```python
from build123d import *

# Parameters (mm, degrees)
F1_DEPTH  = 500
F2_W      = 73.9309489727
F2_H      = 500
F2_H_2    = 305.1662445068
F2_H_3    = 304.9542307854
F3_DEPTH  = 25.4
F4_R      = 5.11898469
F5_DEPTH  = 50.8
F6_R      = 82.2041903744
F6_R_2    = 5.11898469
F7_DEPTH  = 25.4
F8_R      = 5.8344538593
F9_DEPTH  = 50.8
F10_R     = 76.2
F11_DEPTH = 25.4
F12_R     = 6.35
F13_DEPTH = 50.8
F14_R     = 304.8
F14_R_2   = 6.35
F15_DEPTH = 25.4
F16_R     = 6.35
F17_DEPTH = 50.8


with BuildPart() as f1:
    # F0 (on Front) → F1 (new body)
    with BuildSketch(Plane.XZ):
        Polygon((-775.8201853523, 304.8), (-775.8201853523, 0), (500, 0), (500, 500), (0, 500), align=None)
    extrude(amount=F1_DEPTH)

    # F2 (on face) → F3 (join)
    with BuildSketch(Plane(origin=(0, 0, 0), x_dir=(1, 0, 0), z_dir=(0, 0, -1))):
        with Locations((-436.6519004107, 250)):
            Rectangle(F2_W, F2_H)
        with Locations((-436.6519004107, 652.5831222534)):
            Rectangle(F2_W, F2_H_2)
        with Locations((-436.6519004107, -152.4771153927)):
            Rectangle(F2_W, F2_H_3)
    extrude(amount=F3_DEPTH)

    # F4 (on face) → F5 (join)
    with BuildSketch(Plane.XZ.offset(805.1662445068)):
        with Locations((-437.0749592781, -14.6776270121)):
            Circle(F4_R)
    extrude(amount=F5_DEPTH)

    # F6 (on face) → F7 (join)
    with BuildSketch(Plane.XZ.offset(855.9662445068)):
        with Locations((-437.0749592781, -14.6776270121)):
            Circle(F6_R)
        with Locations((-437.0749592781, -14.6776270121)):
            Circle(F6_R_2, mode=Mode.SUBTRACT)
    extrude(amount=-F7_DEPTH)

    # F8 (on face) → F9 (join)
    with BuildSketch(Plane(origin=(0, 304.9542307854, 0), x_dir=(-1, 0, 0), z_dir=(0, 1, 0))):
        with Locations((435.6042742729, -14.3710989505)):
            Circle(F8_R)
    extrude(amount=F9_DEPTH)

    # F10 (on face) → F11 (join)
    with BuildSketch(Plane(origin=(0, 355.7542307854, 0), x_dir=(-1, 0, 0), z_dir=(0, 1, 0))):
        with Locations((435.6042742729, -14.3710989505)):
            Circle(F10_R)
    extrude(amount=-F11_DEPTH)

    # F12 (on face) → F13 (join)
    with BuildSketch(Plane.XZ):
        with Locations((195.2, 152.4)):
            Circle(F12_R)
    extrude(amount=-F13_DEPTH)

    # F14 (on face) → F15 (join)
    with BuildSketch(Plane(origin=(0, 50.8, 0), x_dir=(-1, 0, 0), z_dir=(0, 1, 0))):
        with Locations((-195.2, 152.4)):
            Circle(F14_R)
        with Locations((-195.2, 152.4)):
            Circle(F14_R_2, mode=Mode.SUBTRACT)
    extrude(amount=-F15_DEPTH)

    # F16 (on face) → F17 (join)
    with BuildSketch(Plane.XZ.offset(500)):
        with Locations((210.5554491282, 151.9356071949)):
            Circle(F16_R)
    extrude(amount=F17_DEPTH)


solid = f1.part
```
Read the model definition and answer for the solid it produces. Units are mm, in the model's axes. A direction names the side the tool comes from. Coordinates: 2 decimals unless noted, no trailing zeros. Loops run counter-clockwise (first coordinate to the right, second up) from the corner with the lowest first, then second, coordinate; pieces in that order, holes last.
(1) Flat-ended cylindrical pins translate along their axes: pin 1 Ø6 at (x, y) = (-65, -146) entering from -Z; pin 2 Ø4 at (x, z) = (208.5, 153.5) entering from -Y; pin 3 Ø12.5 at (y, z) = (15, -18.5) entering from +X. Find the tip coordinate at first contact, or state that the pin passes through.
Solution:
pin 1: stops at z = 0
pin 2: stops at y = -550.8
pin 3: stops at x = -399.69
(2) A tool of negligible diameter and unlimited length cuts with its end or side. For faces 1 (the face through (-508.285, 343.232, 8.517)), 2 (the face through (500, -246, 247)), 3 (the face through (-437, -655, 0)), 4 (the face through (-502.31, -843.44, -64.7)), from which of +Z, -Z, +X, -X, +Y, -Y can it reach the whole face along a straight path? Write none if from no direction.
Solution:
face 1: +Y
face 2: +Z, -Z, +X, +Y, -Y
face 3: +Z, +X, -X
face 4: -Y
(3) The part is cut by section D-D (y = -721). Determine the outline of the cut face in (x, z), and give its area (3 significant figures).
Solution:
outline: (-473.62, -25.4) - (-399.69, -25.4) - (-399.69, 0) - (-473.62, 0) - close
area: 1,880 mm2
(4) The part is cut by section A-A (z = 206.5). Determine the outline of the cut face in (x, y), and give its area (3 significant figures).
Solution:
outline: (-775.82, -500) - (500, -500) - (500, 0) - (-775.82, 0) - close; (-104.76, 25.4) - (495.16, 25.4) - (495.16, 50.8) - (-104.76, 50.8) - close
area: 653,000 mm2
(5) The part is cut by section B-B (x = 328.5). Determine the outline of the cut face in (y, z), and give its area (3 significant figures).
Solution:
outline: (-500, 0) - (0, 0) - (0, 500) - (-500, 500) - close; (25.4, -121.71) - (50.8, -121.71) - (50.8, 426.51) - (25.4, 426.51) - close
area: 264,000 mm2
(6) Consider line 1 along Y through (x, z) = (-215.5, 14.5); line 2 along Z through (x, y) = (-465, -501); line 3 along X through (y, z) = (15.5, -13). Determine where each line is inside the solid, lowest interval first.
Solution:
line 1: y = -500 to 0
line 2: z = -25.4 to 0
line 3: x = -473.62 to -399.69
(7) The part is cut by section C-C (z = -55). Determine the outline of the cut face in (x, y).
Solution:
outline: (-508.71, -855.97) - (-365.44, -855.97) - (-365.44, -830.57) - (-508.71, -830.57) - close; (-500.07, 330.35) - (-371.14, 330.35) - (-371.14, 355.75) - (-500.07, 355.75) - close; (-28.16, 25.4) - (418.56, 25.4) - (418.56, 50.8) - (-28.16, 50.8) - close
(8) The mould has two halves that part along Y. Classify faces 5 (the face through (-775.82, -246, 155)), 6 (the face through (-147, 0, 254)), 7 (the face through (199, 50.8, 157)): released by +Y, released by -Y, zero draft, split by the parting line, or undercut.
Solution:
face 5: zero draft
face 6: undercut
face 7: released by +Y
